Verification items for the finished model (mm, model axes). Face numbers are marked on the shaded views. A direction names the side the tool comes from. Give positions to 0.01 mm unless a question says otherwise; leave off trailing zeros. Write each loop counter-clockwise with the first axis right and the second up, starting at its lowest first coordinate (ties: lowest second). Pieces come first, ordered by that corner, then holes. Notation, with made-up numbers: (60.5, 5.25) - (103.5, 5.25) arc R13 ccw to (103.5, 26.25) - close; hole circle Ø11 at (54.25, -24). An arc over 180 degrees is marked (long way). Put each result on its own line as item: value.
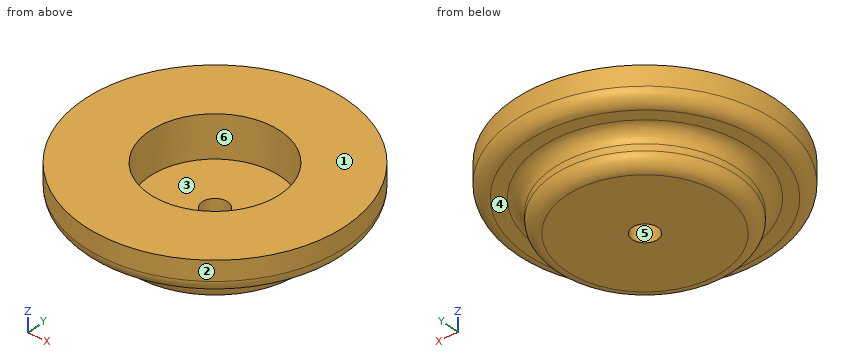
from build123d import *

# Parameters (mm, degrees)
FILLET1_R                        = 2.54
F_10_0_1935_DIAMETER_HOLE1_D     = 4.9149
F_10_0_1935_DIAMETER_HOLE1_DEPTH = 10.16
F_10_0_1935_DIAMETER_HOLE1_TIP   = 1.476584928


with BuildPart() as part:
    # Sketch1 → Revolve1 (revolve)
    with BuildSketch(Plane(origin=(0, 0, 0), x_dir=(0, 0, -1), z_dir=(1, 0, 0)), mode=Mode.PRIVATE) as revolve1_sk:
        Polygon((79.248, 12.7), (79.248, 25.4), (85.598, 25.4), (85.598, 17.78), (91.948, 17.78), (91.948, 0), (87.376, 0), (87.376, 12.7), align=None)
    revolve(revolve1_sk.sketch.rotate(Axis((0, 0, 0), (0, 0, -1)), 90), axis=Axis((0, 0, 0), (0, 0, -1)))

    # Fillet1
    fillet1_edges = [part.edges().sort_by_distance(p)[0] for p in [
        (-17.78, 0, -91.948),
        (-17.78, 0, -85.598),
        (-25.4, 0, -85.598),
    ]]
    fillet(fillet1_edges, radius=FILLET1_R)

    # #10 (0.1935) Diameter Hole1
    with Locations(Plane(origin=(0, 0, -91.948), x_dir=(-1, 0, 0), z_dir=(0, 0, -1))):
        with Locations((0, 0)):
            Hole(F_10_0_1935_DIAMETER_HOLE1_D / 2, depth=F_10_0_1935_DIAMETER_HOLE1_DEPTH)
            with Locations((0, 0, -(F_10_0_1935_DIAMETER_HOLE1_DEPTH + F_10_0_1935_DIAMETER_HOLE1_TIP / 2))):  # 118° drill point
                Cone(0, F_10_0_1935_DIAMETER_HOLE1_D / 2, F_10_0_1935_DIAMETER_HOLE1_TIP, mode=Mode.SUBTRACT)


solid = part.part
Q1. Set-up check for the marked faces 4, 5 and 6: record each of +Z, -Z, +X, -X, +Y, -Y from which the full face is reachable in a straight line by a thin tool's end or side.
Answers follow:
face 4: -Z
face 5: +Z, -Z
face 6: +Z
Q2. Section check C-C, the plane z = -81. Record the cut outline in (x, y), plus the area to 3 significant figures.
Answers follow:
outline: circle Ø50.8 at (0, 0); hole circle Ø25.4 at (0, 0)
area: 1,520 mm2
Q3. Section check D-D, the plane z = -83.75. Record the cut outline in (x, y), plus the area to 3 significant figures.
Answers follow:
outline: circle Ø50.61 at (0, 0); hole circle Ø25.4 at (0, 0)
area: 1,500 mm2
Q4. Go/stop test with flat-tipped pins: pin 1 Ø7.5 at (x, y) = (1, -1.5) entering from +Z; pin 2 Ø5 at (x, z) = (-18, -85) entering from -Y; pin 3 Ø3 at (x, z) = (-17.5, -82.5) entering from +Y; pin 4 Ø12 at (x, y) = (0.5, 7.5) entering from +Z. Record where each tip stops, or that it passes through.
Answers follow:
pin 1: stops at z = -87.38
pin 2: stops at y = -19.74
pin 3: stops at y = 19.73
pin 4: stops at z = -79.25
Q5. Scan lines: line 1 along Y through (x, z) = (0, -82.5); line 2 along Y through (x, z) = (0, -83.75); line 3 along Z through (x, y) = (7.5, 4). Record each from-to range of solid material in increasing order.
Answers follow:
line 1: y = -25.4 to -12.7, 12.7 to 25.4
line 2: y = -25.3 to -12.7, 12.7 to 25.3
line 3: z = -91.95 to -87.38
Q6. Release check for a two-part mould opening along Y. For the marked faces 1, 2 and 3 record: released by +Y, released by -Y, zero draft, split by the parting line, or undercut.
Answers follow:
face 1: zero draft
face 2: split by the parting line
face 3: undercut
Q7. Section check A-A, the plane y = 0. Record the cut outline in (x, z).
Answers follow:
outline: (-25.4, -83.06) arc R2.54 ccw to (-22.86, -85.6) - (-20.32, -85.6) arc R2.54 cw to (-17.78, -88.14) - (-17.78, -89.41) arc R2.54 ccw to (-15.24, -91.95) - (-2.46, -91.95) - (-2.46, -87.38) - (-12.7, -87.38) - (-12.7, -79.25) - (-25.4, -79.25) - close; (2.46, -91.95) - (15.24, -91.95) arc R2.54 ccw to (17.78, -89.41) - (17.78, -88.14) arc R2.54 cw to (20.32, -85.6) - (22.86, -85.6) arc R2.54 ccw to (25.4, -83.06) - (25.4, -79.25) - (12.7, -79.25) - (12.7, -87.38) - (2.46, -87.38) - close
